from build123d import *

# Parameters (mm, degrees)
BOSS_EXTRUDE1_DEPTH = 57.15
SKETCH2_R           = 19.05
BOSS_EXTRUDE2_DEPTH = 82.55
BOSS_EXTRUDE3_DEPTH = 19.05
SKETCH4_R           = 3.175
CUT_EXTRUDE1_DEPTH  = 154.666273922
BOSS_EXTRUDE4_DEPTH = 222.25
SKETCH6_R           = 10.033
CUT_EXTRUDE2_DEPTH  = 203.2


with BuildPart() as part:
    # Sketch1 → Boss-Extrude1 (new body)
    with BuildSketch(Plane(origin=(0, 0, 0), x_dir=(0, 0, -1), z_dir=(1, 0, 0))):
        with BuildLine():
            Line((-13.589, 19.05), (13.589, 19.05))
            Line((13.589, 19.05), (19.939, 12.7))
            Line((19.939, 12.7), (19.939, -37.211))
            ThreePointArc((19.939, -37.211), (0, -57.15), (-19.939, -37.211))
            Line((-19.939, -37.211), (-19.939, 12.7))
            Line((-19.939, 12.7), (-13.589, 19.05))
        make_face()
    extrude(amount=BOSS_EXTRUDE1_DEPTH)

    # Sketch2 → Boss-Extrude2 (add)
    with BuildSketch(Plane(origin=(57.15, 0, 0), x_dir=(0, 0, -1), z_dir=(1, 0, 0))):
        with Locations((0, -37.211)):
            Circle(SKETCH2_R)
    extrude(amount=BOSS_EXTRUDE2_DEPTH)

    # Sketch3 → Boss-Extrude3 (add)
    with BuildSketch(Plane.ZY):
        Polygon((-6.35, 8.89), (6.35, 8.89), (8.89, 6.35), (8.89, -6.35), (6.35, -8.89), (-6.35, -8.89), (-8.89, -6.35), (-8.89, 6.35), align=None)
    extrude(amount=BOSS_EXTRUDE3_DEPTH)

    # Sketch4 → Cut-Extrude1 (cut, through all)
    with BuildSketch(Plane.XY.offset(8.89)):
        with Locations((-11.684, 0)):
            Circle(SKETCH4_R)
    extrude(amount=-CUT_EXTRUDE1_DEPTH, mode=Mode.SUBTRACT)

    # Sketch5 → Boss-Extrude4 (add)
    with BuildSketch(Plane(origin=(57.15, 0, 0), x_dir=(0, 0, -1), z_dir=(1, 0, 0))):
        with BuildLine():
            Line((-13.589, 19.05), (13.589, 19.05))
            Line((13.589, 19.05), (17.255800165, 4.285529215))
            ThreePointArc((17.255800165, 4.285529215), (0, -17.78), (-17.255800165, 4.285529215))
            Line((-17.255800165, 4.285529215), (-13.589, 19.05))
        make_face()
    extrude(amount=BOSS_EXTRUDE4_DEPTH)

    # Sketch6 → Cut-Extrude2 (cut)
    with BuildSketch(Plane(origin=(279.4, 0, 0), x_dir=(0, 0, -1), z_dir=(1, 0, 0))):
        Circle(SKETCH6_R)
    extrude(amount=-CUT_EXTRUDE2_DEPTH, mode=Mode.SUBTRACT)


solid = part.part
The model under review builds one solid part; all positions refer to its coordinate system, in mm. A direction names the side the tool comes from. Coordinates: 2 decimals unless noted, no trailing zeros. Loops run counter-clockwise (first coordinate to the right, second up) from the corner with the lowest first, then second, coordinate; pieces in that order, holes last. Notation, with made-up numbers: M 75,62 L 86,62 A35 ccw 86,97 Z; hole C -1,81 d2. An arc over 180 degrees is marked long. Put each result on its own line as item: value. Start each with the question number.
Q1. Clearance check with flat-ended pins moving along their axes: pin 1 (14 mm diameter, centred on x = -10, z = -3, fed in from +Y); pin 2 (7.5 mm diameter, centred on x = -11.684, y = 0, fed in from +Z); pin 3 (10 mm diameter, centred on y = 3.5, z = 14.5, fed in from -X). State where each tip first meets the part, or that it passes through.
Q2. Add section A-A (x = 113). Write out the cut boundary in (y, z), and give its area (3 significant figures).
Q3. Add section C-C (y = 0). Write out the cut boundary in (x, z).
Q4. For faces 1 (the flat face through (-9, -8.89, 0)), 2 (the flat face through (166.72, 11.56, 15.45)), 3 (the flat face through (-9, 8.89, 0)), 4 (the flat face through (-7, 0, -8.89)), 5 (the cylindrical face through (166.719, -17.774, -0.452)), list the 3-axis set-ups (+Z, -Z, +X, -X, +Y, -Y) from which the entire face can be reached by the end or side of a thin tool; tool diameter is ignored.
Q5. Wall thickness on line 1 (Y direction, x = 103, z = 0.5); line 2 (Y direction, x = 48, z = 0.5); line 3 (X direction, y = -18, z = 16.5): over which ranges is each line inside the solid? List them lowest first.
Q6. Add section B-B (z = 0). Write out the cut boundary in (x, y) (3 decimals), and give its area (3 significant figures).
Q7. Add section D-D (x = 23). Write out the cut boundary in (y, z).
Q8. The part is to be moulded in two halves that separate along Z. For faces 6 (the flat face through (-7, 0, 8.89)), 7 (the flat face through (166.719, 11.771, -15.397)), 8 (the flat face through (76.2, 0, 0)), say which applies: +Z half, -Z half, draft (parallel to the pull), parting line (faces both ways), or undercut.
Answers:
1. pin 1: stops at y = 8.89
1. pin 2: stops at z = 8.89
1. pin 3: stops at x = 0
2. outline: C -37.21,0 d38.1; M 4.29,-17.26 L 19.05,-13.59 L 19.05,13.59 L 4.29,17.26 A17.78 ccw long Z; hole C 0,0 d20.07
2. area: 1,930 mm^2
3. outline: M -19.05,-8.89 L -14.86,-8.89 L -14.86,8.89 L -19.05,8.89 Z; M -8.51,-8.89 L 0,-8.89 L 0,-19.94 L 57.15,-19.94 L 57.15,-17.78 L 279.4,-17.78 L 279.4,-10.03 L 76.2,-10.03 L 76.2,10.03 L 279.4,10.03 L 279.4,17.78 L 57.15,17.78 L 57.15,19.94 L 0,19.94 L 0,8.89 L -8.51,8.89 Z
4. face 1: +Z, -Z, -X, -Y
4. face 2: +Z, +X, +Y
4. face 3: +Z, -Z, -X, +Y
4. face 4: -Z, -X, +Y, -Y
4. face 5: +X
5. line 1: y = -56.25 to -18.17, -17.77 to -10.02, 10.02 to 19.05
5. line 2: y = -57.14 to 19.05
5. line 3: x = 0 to 57.15
6. outline: M -19.05,-8.89 L 0,-8.89 L 0,-57.15 L 57.15,-57.15 L 57.15,-56.261 L 139.7,-56.261 L 139.7,-18.161 L 57.15,-18.161 L 57.15,-17.78 L 279.4,-17.78 L 279.4,-10.033 L 76.2,-10.033 L 76.2,10.033 L 279.4,10.033 L 279.4,19.05 L 0,19.05 L 0,8.89 L -19.05,8.89 Z; hole C -11.684,0 d6.35
6. area: 11,900 mm^2
7. outline: M -37.21,-19.94 L 12.7,-19.94 L 19.05,-13.59 L 19.05,13.59 L 12.7,19.94 L -37.21,19.94 A19.94 ccw Z
8. face 6: +Z half
8. face 7: -Z half
8. face 8: undercut
